```python
from build123d import *

# Parameters (mm, degrees)
SKETCH1_R           = 1.3
BOSS_EXTRUDE1_DEPTH = 2.54
FILLET1_R           = 1.016


with BuildPart() as part:
    # Sketch1 → Boss-Extrude1 (new body)
    with BuildSketch(Plane(origin=(0, 0, 0), x_dir=(1, 0, 0), z_dir=(0, 1, 0))):
        with BuildLine():
            Line((0, 3.556), (33.02, 3.556))
            ThreePointArc((33.02, 3.556), (36.576, 0), (33.02, -3.556))
            Line((33.02, -3.556), (0, -3.556))
            ThreePointArc((0, -3.556), (-3.556, 0), (0, 3.556))
        make_face()
        with Locations(Location((0, 0, 0), (0, 0, 270))):
            Circle(SKETCH1_R, mode=Mode.SUBTRACT)
        with Locations(Location((33.02, 0, 0), (0, 0, 270))):
            Circle(SKETCH1_R, mode=Mode.SUBTRACT)
    extrude(amount=BOSS_EXTRUDE1_DEPTH)

    # Fillet1
    fillet1_edges = [part.edges().sort_by_distance(p)[0] for p in [
        (36.576, 2.54, 0),
        (16.51, 2.54, -3.556),
        (-3.556, 2.54, 0),
        (16.51, 2.54, 3.556),
    ]]
    fillet(fillet1_edges, radius=FILLET1_R)


solid = part.part
```
Can you work these out from the model? Positions are in its coordinate system, mm. Coordinates: 2 decimals unless noted, no trailing zeros. Order: outer loops, then holes, each group sorted by start corner. A loop starts at its lowest first (then second) coordinate and runs counter-clockwise, first axis right, second up. Notation, with made-up numbers: (6, 22) - (57, 22) arc R10 ccw to (57, 33) - close; hole circle Ø8 at (44.25, 34.5). An arc over 180 degrees is marked (long way). Answer in a Markdown table with one row per item.
1. Suppose I cut it at A-A (y = 0.35). Please give me the cut outline in (x, z), and give its area (3 significant figures).
Reply:
| item | result |
|---|---|
| outline | (0, -3.56) - (33.02, -3.56) arc R3.56 ccw to (33.02, 3.56) - (0, 3.56) arc R3.56 ccw to start; hole circle Ø2.6 at (0, 0); hole circle Ø2.6 at (33.02, 0) |
| area | 264 mm^2 |
2. Suppose I cut it at C-C (x = 20). Please give me the cut outline in (y, z).
Reply:
| item | result |
|---|---|
| outline | (0, -3.56) - (1.52, -3.56) arc R1.02 ccw to (2.54, -2.54) - (2.54, 2.54) arc R1.02 ccw to (1.52, 3.56) - (0, 3.56) - close |
3. If we mould it in two halves opening along Z, with no side actions, what happens to faces 1 (the flat face through (17, 0, 0)), 2 (the flat face through (16, 1, -3.556)), 3 (the cylindrical face through (34.116, 1.252, 0.699)), 4 (the cylindrical face through (0.39, 1.25, 1.24))? For each: pulls with the +Z half, pulls with the -Z half, needs draft (parallel to the pull), parting line crosses it, or undercut.
Reply:
| item | result |
|---|---|
| face 1 | needs draft |
| face 2 | pulls with the -Z half |
| face 3 | undercut |
| face 4 | undercut |
4. For pin 1 (2 mm diameter, centred on x = 12.5, z = -2, fed in from -Y); pin 2 (1.5 mm diameter, centred on y = 1.5, z = -2, fed in from +X), each with a flat end and sliding along its axis, tell me the tip position at first contact or that it passes through.
Reply:
| item | result |
|---|---|
| pin 1 | stops at y = 0 |
| pin 2 | stops at x = 36.35 |
5. Suppose I cut it at B-B (z = 0). Please give me the cut outline in (x, y), and give its area (3 significant figures).
Reply:
| item | result |
|---|---|
| outline | (-3.56, 0) - (-1.3, 0) - (-1.3, 2.54) - (-2.54, 2.54) arc R1.02 ccw to (-3.56, 1.52) - close; (1.3, 0) - (31.72, 0) - (31.72, 2.54) - (1.3, 2.54) - close; (34.32, 0) - (36.58, 0) - (36.58, 1.52) arc R1.02 ccw to (35.56, 2.54) - (34.32, 2.54) - close |
| area | 88.3 mm^2 |
6. If I drill on line 1 along X through (y, z) = (1.6, 0); line 2 along Z through (x, y) = (-1, 0.95), over which ranges is the centre line in solid material (lowest first)?
Reply:
| item | result |
|---|---|
| line 1 | x = -3.55 to -1.3, 1.3 to 31.72, 34.32 to 36.57 |
| line 2 | z = -3.41 to -0.83, 0.83 to 3.41 |
